from build123d import *

# Parameters (mm, degrees)
SKETCH1_R           = 7.5
BOSS_EXTRUDE2_DEPTH = 10
FILLET1_R           = 10


with BuildPart() as part:
    # Sketch1 → Boss-Extrude2 (new body)
    with BuildSketch(Plane.XY):
        with BuildLine():
            add(Edge.make_bspline(
                [(20, 0), (20.020409748, 0.037996513), (20.060928024, 0.114187014), (20.12964942, 0.245531013), (20.227524178, 0.436799942), (20.320803466, 0.624005393), (20.408101904, 0.80454476), (20.513131341, 1.028153853), (20.636379782, 1.30013819), (20.775890348, 1.622275603), (20.964561763, 2.084363584), (21.176160839, 2.645597494), (21.400762948, 3.308060339), (21.627348817, 4.074879511), (21.82387956, 4.849852237), (21.990628499, 5.631814908), (22.127804945, 6.419471307), (22.343605386, 8.00388274), (22.444295112, 10.004224504), (22.324306643, 12.205875028), (21.865414458, 14.9688026), (21.194781507, 17.482815576), (20.196975773, 20.103806606), (18.711348901, 22.943135572), (16.913850005, 25.595374807), (14.83803254, 28.035320632), (12.481825943, 30.276438116), (9.905551794, 32.260621181), (7.143058118, 33.975373516), (3.508895363, 35.76599482), (-1.037505048, 37.342198382), (-5.776049389, 38.226758726), (-10.58060247, 38.430948462), (-14.572645562, 38.161653345), (-17.738378195, 37.689516547), (-20.856812898, 36.968897142), (-23.909970253, 36.009023208), (-26.881276298, 34.820013511), (-29.755513368, 33.41273371), (-32.518812511, 31.798646577), (-34.82859609, 30.215871445), (-36.724133372, 28.745155323), (-38.244357448, 27.447549659), (-39.423774282, 26.367755023), (-40.565156508, 25.248103031), (-41.667740599, 24.089758356), (-42.597224858, 23.04452492), (-43.368854904, 22.125890975), (-44.11890301, 21.191619014), (-44.849652331, 20.238158336), (-45.491908008, 19.351069223), (-46.0606176, 18.522333813), (-46.44278908, 17.945992785), (-46.663264674, 17.607165405), (-46.845252854, 17.321947665), (-46.938757793, 17.174061248), (-46.984631039, 17.101007167)],
                knots=[0.050324208, 0.050324208, 0.050324208, 0.050324208, 0.050324208, 0.052007215, 0.053690221, 0.055373228, 0.057056234, 0.058739241, 0.060422248, 0.063788261, 0.067154274, 0.070520287, 0.077252313, 0.083984355, 0.090716396, 0.097448438, 0.10418048, 0.110912521, 0.117644561, 0.151304782, 0.171500944, 0.184965059, 0.211893341, 0.238821591, 0.265749806, 0.292678076, 0.319606256, 0.346534414, 0.375101607, 0.402029829, 0.428958051, 0.48281442, 0.536670848, 0.563599055, 0.590527261, 0.61745547, 0.644383679, 0.671311911, 0.698240144, 0.725168325, 0.752096507, 0.779024722, 0.79248883, 0.805952937, 0.819417041, 0.832881144, 0.846345248, 0.859809351, 0.866541414, 0.873273478, 0.886737604, 0.900201731, 0.903567763, 0.906933794, 0.910299826, 0.913665858, 0.913665858, 0.913665858, 0.913665858, 0.913665858], degree=4))
            add(Edge.make_bspline(
                [(-46.984631039, 17.101007167), (-47.008245687, 16.930252773), (-47.052453505, 16.594747959), (-47.14772288, 15.834487365), (-47.214528259, 15.160715188), (-47.293965593, 14.299779503), (-47.346314657, 13.538629173), (-47.392988991, 12.722186285), (-47.422468156, 11.933538608), (-47.444946495, 10.930726825), (-47.444010053, 9.735376393), (-47.404361039, 8.336368598), (-47.304511764, 6.742720001), (-47.111846077, 4.754565727), (-46.771162846, 2.38206492), (-46.213481433, -0.359572326), (-45.355872486, -3.439660234), (-44.413431344, -6.073991193), (-43.469633124, -8.277605724), (-42.593502891, -10.072305051), (-41.839303321, -11.480778659), (-40.830669548, -13.204502076), (-39.516241362, -15.209384647), (-37.834348338, -17.445666738), (-35.716475971, -19.841921409), (-32.836422898, -22.614479765), (-29.03089004, -25.547737865), (-24.838756286, -27.918909191), (-20.349017446, -29.638470379), (-16.397837157, -30.613103542), (-13.160898489, -31.080464427), (-9.892857606, -31.217237714), (-6.628606497, -31.010938023), (-3.473189469, -30.47401424), (-0.394676097, -29.596112443), (2.565112202, -28.37500671), (5.36075444, -26.812990946), (7.781768771, -25.036326324), (9.9742179, -22.985943497), (11.63958792, -20.986683376), (12.748810807, -19.3214148), (13.515819977, -17.919279199), (13.906378968, -17.109859569), (14.149100741, -16.562152771), (14.339295058, -16.100610712), (14.484089284, -15.728391771), (14.621373048, -15.353433154), (14.751011091, -14.975917501), (14.873112977, -14.594855978), (14.987276237, -14.211724793), (15.091962981, -13.833461004), (15.191298738, -13.439798185), (15.266942281, -13.107906017), (15.303325903, -12.940133069), (15.320888863, -12.855752194)],
                knots=[0.086334142, 0.086334142, 0.086334142, 0.086334142, 0.086334142, 0.093060515, 0.099786888, 0.10651326, 0.113239633, 0.119966006, 0.126692378, 0.133418751, 0.140145123, 0.153597846, 0.167050569, 0.180503291, 0.193956014, 0.220861466, 0.247766918, 0.274672338, 0.301577759, 0.315030493, 0.328483227, 0.341935962, 0.355388696, 0.382294142, 0.409199588, 0.436105031, 0.463010473, 0.516821378, 0.570632207, 0.597537677, 0.624443147, 0.653716038, 0.680621422, 0.707526854, 0.734432293, 0.761337694, 0.788243181, 0.815148711, 0.842054217, 0.862233312, 0.889138718, 0.902591415, 0.909317764, 0.916044113, 0.919407288, 0.922770462, 0.926133629, 0.929496795, 0.932859961, 0.936223127, 0.939586294, 0.94294946, 0.946312626, 0.949675792, 0.949675792, 0.949675792, 0.949675792, 0.949675792], degree=4))
            add(Edge.make_bspline(
                [(15.320888863, -12.855752194), (15.365482074, -12.802608074), (15.453982567, -12.695704505), (15.663171852, -12.439954999), (15.827525813, -12.226893605), (16.052433323, -11.933079522), (16.234262328, -11.682018392), (16.434764749, -11.400135846), (16.616884894, -11.131589611), (16.802556699, -10.850279333), (16.979014347, -10.571395037), (17.196540035, -10.215824071), (17.44658158, -9.785182904), (17.725195173, -9.273842637), (18.023456431, -8.679695549), (18.302106839, -8.075852302), (18.560352889, -7.462892724), (18.798195449, -6.842210014), (19.015199451, -6.212979877), (19.211229439, -5.578581169), (19.386005403, -4.935179764), (19.539372739, -4.291022665), (19.671138501, -3.634366779), (19.781171398, -2.986524336), (19.869341032, -2.3139722), (19.935555478, -1.675574724), (19.974215132, -1.055908566), (19.993553165, -0.61958797), (19.999079015, -0.206445905), (20, -0.069374722), (20, 0)],
                knots=[0.08263773, 0.08263773, 0.08263773, 0.08263773, 0.08263773, 0.102512123, 0.122386517, 0.142260911, 0.162135305, 0.182009699, 0.201884093, 0.221758486, 0.24163288, 0.261507274, 0.281381668, 0.321130456, 0.360879243, 0.400628031, 0.440376819, 0.480125606, 0.519874394, 0.559623181, 0.599371969, 0.639120757, 0.678869544, 0.718618332, 0.75836712, 0.798115907, 0.837864695, 0.877613483, 0.897487877, 0.91736227, 0.91736227, 0.91736227, 0.91736227, 0.91736227], degree=4))
        make_face()
        Circle(SKETCH1_R, mode=Mode.SUBTRACT)
    extrude(amount=BOSS_EXTRUDE2_DEPTH)

    # Fillet1
    fillet1_edges = [part.edges().sort_by_distance(p)[0] for p in [
        (-46.984631039, 17.101007167, 5),
        (15.320888863, -12.855752194, 5),
        (20, 0, 5),
    ]]
    fillet(fillet1_edges, radius=FILLET1_R)


solid = part.part
Here's how the part is built. I have some questions about the finished solid (model axes, mm). Give positions to 0.01 mm unless a question says otherwise; leave off trailing zeros. Use a Markdown table: item, result. Add a question column.
Item 1: Will these pins go through, and if not, where does the flat tip stop? pin 1 (5 mm diameter, centred on y = -6.5, z = 8, fed in from -X); pin 2 (3 mm diameter, centred on y = 16.5, z = 3.5, fed in from +X); pin 3 (1 mm diameter, centred on x = -40, y = -17, fed in from +Z).
Item 2: If we mould it in two halves opening along Y, with no side actions, what happens to faces 1 (the face through (-13, 4, 0)), 2 (the face through (-7.493, 0.33, 4.93))? For each: pulls with the +Y half, pulls with the -Y half, needs draft (parallel to the pull), parting line crosses it, or undercut.
Item 3: I need wall thicknesses on line 1 (X direction, y = 5, z = 6); line 2 (Y direction, x = 0, z = 3.5) (3 decimals); line 3 (X direction, y = 4, z = 1). Which ranges of each line are inside material? Lowest first, please.
Data:
| question | item | result |
|---|---|---|
| 1 | pin 1 | stops at x = -45.12 |
| 1 | pin 2 | stops at x = 21.81 |
| 1 | pin 3 | passes through |
| 2 | face 1 | needs draft |
| 2 | face 2 | undercut |
| 3 | line 1 | x = -47.12 to -5.59, 5.59 to 21.85 |
| 3 | line 2 | y = -29.375 to -7.5, 7.5 to 36.875 |
| 3 | line 3 | x = -46.99 to -6.34, 6.34 to 21.6 |
